from build123d import *

# Parameters (mm, degrees)
ESBO_O1_W       = 18.5
ESBO_O1_H       = 39
EXTRUS_O1_DEPTH = 1.5
EXTRUS_O2_DEPTH = 8
ESBO_O3_W       = 18.5
ESBO_O3_H       = 1.5
EXTRUS_O3_DEPTH = 24.580977503


with BuildPart() as part:
    # Esboço1 → Extrusão1 (new body)
    with BuildSketch(Plane(origin=(0, 0, 0), x_dir=(1, 0, 0), z_dir=(0, 1, 0))):
        Rectangle(ESBO_O1_W, ESBO_O1_H)
    extrude(amount=EXTRUS_O1_DEPTH)

    # Esboço2 → Extrusão2 (add)
    with BuildSketch(Plane(origin=(0, 1.5, 0), x_dir=(1, 0, 0), z_dir=(0, 1, 0))):
        Polygon((7.75, 19.5), (9.25, 19.5), (9.25, -19.5), (-9.25, -19.5), (-9.25, 19.5), (-7.75, 19.5), (-7.75, -18), (7.75, -18), align=None)
    extrude(amount=EXTRUS_O2_DEPTH)

    # Esboço3 → Extrusão3 (cut, through all)
    with BuildSketch(Plane(origin=(0, 9.5, 0), x_dir=(1, 0, 0), z_dir=(0, 1, 0))):
        with Locations((0, -18.75)):
            Rectangle(ESBO_O3_W, ESBO_O3_H)
    extrude(amount=-EXTRUS_O3_DEPTH, mode=Mode.SUBTRACT)


solid = part.part
Here's how the part is built. I have some questions about the finished solid (model axes, mm). A direction names the side the tool comes from. Round coordinates to 2 decimals unless told otherwise and drop trailing zeros. Write each loop counter-clockwise with the first axis right and the second up, starting at its lowest first coordinate (ties: lowest second). Pieces come first, ordered by that corner, then holes.
1. Suppose I cut it at A-A (z = 4). List the corners of the cut face in (x, y) for me.
2. If we mould it in two halves opening along X, with no side actions, what happens to faces 3 (the flat face through (0, 0, -1)), 4 (the flat face through (7.75, 5, 0)), 5 (the flat face through (9.25, 5, -1))? For each: released by +X, released by -X, zero draft, split by the parting line, or undercut.
3. Suppose I cut it at B-B (y = 6.5). List the corners of the cut face in (x, z) for me.
4. For faces 1 (the flat face through (-8, 9.5, -1)), 2 (the flat face through (-7.75, 5, -1)), which set-ups out of +Z, -Z, +X, -X, +Y, -Y let a thin tool reach every point of the face, with its end or its side?
5. I need wall thicknesses on L1, parallel to X at y = 3.75, z = -13; L2, parallel to Y at x = 4, z = -3.5. Which ranges of each line are inside material? Lowest first, please.
6. Will these pins go through, and if not, where does the flat tip stop? pin 1 Ø4 at (x, z) = (-5, -12.5) entering from +Y; pin 2 Ø5 at (x, y) = (3.5, 8) entering from -Z.
7. Suppose I cut it at C-C (x = 1.5). List the corners of the cut face in (y, z) for me, and give its area (4 significant figures).
Answer sheet:
1. outline: (-9.25, 0) - (9.25, 0) - (9.25, 9.5) - (7.75, 9.5) - (7.75, 1.5) - (-7.75, 1.5) - (-7.75, 9.5) - (-9.25, 9.5) - close
2. face 3: zero draft
2. face 4: undercut
2. face 5: released by +X
3. outline: (-9.25, -19.5) - (-7.75, -19.5) - (-7.75, 18) - (-9.25, 18) - close; (7.75, -19.5) - (9.25, -19.5) - (9.25, 18) - (7.75, 18) - close
4. face 1: +Z, -Z, +X, -X, +Y
4. face 2: +Z, -Z, +Y
5. L1: x = -9.25 to -7.75, 7.75 to 9.25
5. L2: y = 0 to 1.5
6. pin 1: stops at y = 1.5
6. pin 2: passes through
7. outline: (0, -19.5) - (1.5, -19.5) - (1.5, 18) - (0, 18) - close
7. area: 56.25 mm2
